Here's how the part is built. I have some questions about the finished solid (model axes, mm). Face numbers are marked on the shaded views. A direction names the side the tool comes from. Round coordinates to 2 decimals unless told otherwise and drop trailing zeros. Write each loop counter-clockwise with the first axis right and the second up, starting at its lowest first coordinate (ties: lowest second). Pieces come first, ordered by that corner, then holes. Notation, with made-up numbers: (38.5, 62) -> (72.5, 62) arc R23 ccw to (72.5, 78) -> close; hole circle Ø5 at (-5, 37.5). An arc over 180 degrees is marked (long way). Answer as CSV lines item,"result".
```python
from build123d import *

# Parameters (mm, degrees)
F1_DEPTH    = 10
F3_DEPTH    = 48
F4_T1_DEPTH = 30
F5_T1_DEPTH = 30
F6_R        = 6
F7_DEPTH    = 3
F8_W        = 28
F8_H        = 5
F9_DEPTH    = 2
F10_DEPTH   = 25


# Not quite as in the source:
# - a fillet or chamfer that OpenCascade refuses, or shapes differently, is made with other operations: its cross-section is extruded or revolved along the edge and cut away or added


with BuildPart() as f1:
    # F0 (on Top) → F1 (new body)
    with BuildSketch(Plane.XY):
        with BuildLine():
            Line((-15, 30), (-46, 30))
            Line((-46, 30), (-46, -12))
            ThreePointArc((-46, -12), (-44.2426406871, -16.2426406871), (-40, -18))
            Line((-40, -18), (40, -18))
            ThreePointArc((40, -18), (44.2426406871, -16.2426406871), (46, -12))
            Line((46, -12), (46, 30))
            Line((46, 30), (15, 30))
            Line((15, 30), (15, 10))
            Line((15, 10), (-15, 10))
            Line((-15, 10), (-15, 30))
        make_face()
    extrude(amount=F1_DEPTH)

    # F2 (on Top) → F3 (join)
    with BuildSketch(Plane.XY):
        Polygon((-15, 30), (-25, 30), (-25, 0), (25, 0), (25, 30), (15, 30), (15, 10), (-15, 10), align=None)
    extrude(amount=F3_DEPTH)

    # F4: fillet of radius 25 on 1 edges, made by hand

    # F4_s2 → F4_t1 (join)
    with BuildSketch(Plane.XZ.offset(-30)):
        with BuildLine():
            ThreePointArc((-46, 10), (-30.9605672353, 18.4760736125), (-25, 34.6779253585))
            Line((-25, 34.6779253585), (-25, 10))
            Line((-25, 10), (-46, 10))
        make_face()
    extrude(amount=F4_T1_DEPTH)

    # F5: fillet of radius 25 on 1 edges, made by hand

    # F5_s2 → F5_t1 (join)
    with BuildSketch(Plane.XZ.offset(-30)):
        with BuildLine():
            ThreePointArc((46, 10), (30.9605672353, 18.4760736125), (25, 34.6779253585))
            Line((25, 34.6779253585), (25, 10))
            Line((25, 10), (46, 10))
        make_face()
    extrude(amount=F5_T1_DEPTH)

    # F6 (on face) → F7 (join)
    with BuildSketch(Plane.XZ):
        with BuildLine():
            Line((14, 10), (14, 29))
            ThreePointArc((14, 29), (0, 43), (-14, 29))
            Line((-14, 29), (-14, 10))
            Line((-14, 10), (14, 10))
        make_face()
        with Locations((0, 29)):
            Circle(F6_R, mode=Mode.SUBTRACT)
    extrude(amount=F7_DEPTH)

    # F8 (on face) → F9 (join)
    with BuildSketch(Plane.XZ.offset(3)):
        with Locations((0, 12.5)):
            Rectangle(F8_W, F8_H)
    extrude(amount=F9_DEPTH)

    # F10 (cut): a face of the model
    f10_faces = [f1.faces().sort_by_distance(p)[0] for p in [
        (0, 0, 29),
    ]]
    extrude(f10_faces, amount=-F10_DEPTH, mode=Mode.SUBTRACT)


solid = f1.part
```
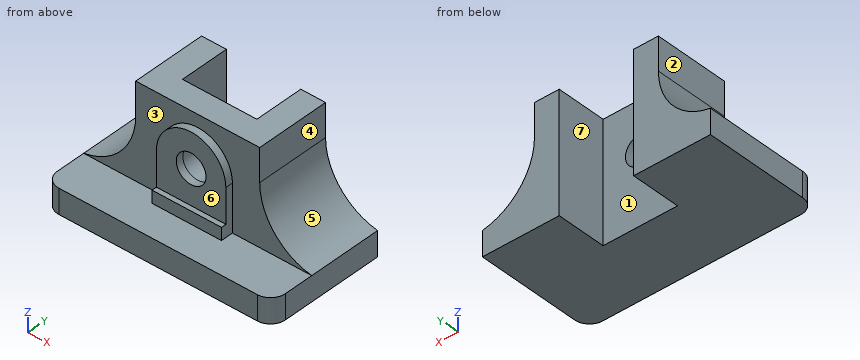
1. Suppose I cut it at D-D on z = 17.5. Please give me the cut outline in (x, y).
Numbers:
outline,"(-31.84, 0) -> (-14, 0) -> (-14, -3) -> (14, -3) -> (14, 0) -> (31.84, 0) -> (31.84, 30) -> (15, 30) -> (15, 10) -> (-15, 10) -> (-15, 30) -> (-31.84, 30) -> close"
2. Suppose I cut it at B-B on x = 0. Please give me the cut outline in (y, z), and give its area (3 significant figures).
Numbers:
outline,"(-18, 0) -> (10, 0) -> (10, 23) -> (-3, 23) -> (-3, 15) -> (-5, 15) -> (-5, 10) -> (-18, 10) -> close; (-3, 35) -> (10, 35) -> (10, 48) -> (0, 48) -> (0, 43) -> (-3, 43) -> close"
area,"613 mm^2"
3. On a 3-axis mill with a long thin cutter (end or side, diameter ignored), from which of +Z, -Z, +X, -X, +Y, -Y can I reach the whole of each face in a straight line? I mean the marked faces 1, 2, 3 and 4. Say none if no direction works.
Numbers:
face 1,"+Z, -Z, +Y"
face 2,"+Z, -X, +Y, -Y"
face 3,"+Z, -Y"
face 4,"+Z, +X, +Y, -Y"
4. Suppose I cut it at C-C on x = -16. Please give me the cut outline in (y, z).
Numbers:
outline,"(-18, 0) -> (30, 0) -> (30, 48) -> (0, 48) -> (0, 10) -> (-18, 10) -> close"
5. Suppose I cut it at A-A on y = 11.5. Please give me the cut outline in (x, z).
Numbers:
outline,"(-46, 0) -> (-15, 0) -> (-15, 48) -> (-25, 48) -> (-25, 34.68) arc R25 cw to (-46, 10) -> close; (15, 0) -> (46, 0) -> (46, 10) arc R25 cw to (25, 34.68) -> (25, 48) -> (15, 48) -> close"
6. If I drill on line 1 (X direction, y = 15, z = 38.5); line 2 (Z direction, x = 0, y = -1); line 3 (Z direction, x = 0, y = 5.25), over which ranges is the centre line in solid material (lowest first)?
Numbers:
line 1,"x = -25 to -15, 15 to 25"
line 2,"z = 0 to 23, 35 to 43"
line 3,"z = 0 to 23, 35 to 48"
7. For pin 1 Ø15.5 at (x, z) = (0, 29) entering from -Y; pin 2 Ø10 at (y, z) = (23.5, 16.5) entering from +X; pin 3 Ø4 at (y, z) = (-1.5, 23.5) entering from -X; pin 4 Ø1.5 at (y, z) = (-5.5, 29.5) entering from -X, each with a flat end and sliding along its axis, tell me the tip position at first contact or that it passes through.
Numbers:
pin 1,"stops at y = -3"
pin 2,"stops at x = 40.63"
pin 3,"stops at x = -28.35"
pin 4,"passes through"
8. If we mould it in two halves opening along X, with no side actions, what happens to the marked faces 5, 6 and 7? For each: released by +X, released by -X, zero draft, split by the parting line, or undercut.
Numbers:
face 5,"released by +X"
face 6,"zero draft"
face 7,"undercut"
